The model under review builds one solid part; all positions refer to its coordinate system, in mm. A direction names the side the tool comes from. Give positions to 0.01 mm unless a question says otherwise; leave off trailing zeros. Order: outer loops, then holes, each group sorted by start corner. A loop starts at its lowest first (then second) coordinate and runs counter-clockwise, first axis right, second up.
```python
from build123d import *

# Parameters (mm, degrees)
SKETCH1_W                      = 225
SKETCH1_H                      = 150
SKETCH1_W_2                    = 5
SKETCH1_H_2                    = 80
BOSS_EXTRUDE1_DEPTH            = 5
CBORE_FOR_M5_SBHCS1_AT_2_COUNT = 2
CBORE_FOR_M5_SBHCS1_AT_2_PITCH = 210
CBORE_FOR_M5_SBHCS1_AT_3_COUNT = 2
CBORE_FOR_M5_SBHCS1_AT_3_PITCH = 135
CBORE_FOR_M5_SBHCS1_AT_4_COUNT = 2
CBORE_FOR_M5_SBHCS1_AT_4_PITCH = 249.649754656
FILLET1_R                      = 2


with BuildPart() as part:
    # Sketch1 → Boss-Extrude1 (new body)
    with BuildSketch(Plane(origin=(0, 0, 0), x_dir=(1, 0, 0), z_dir=(0, 1, 0))):
        Rectangle(SKETCH1_W, SKETCH1_H)
        with Locations((100, 0)):
            Rectangle(SKETCH1_W_2, SKETCH1_H_2, mode=Mode.SUBTRACT)
        with Locations((90, 0)):
            Rectangle(SKETCH1_W_2, SKETCH1_H_2, mode=Mode.SUBTRACT)
        with Locations((80, 0)):
            Rectangle(SKETCH1_W_2, SKETCH1_H_2, mode=Mode.SUBTRACT)
    extrude(amount=BOSS_EXTRUDE1_DEPTH)

    # Sketch3 → CBORE for M5 SBHCS1 (revolve, cut)
    with BuildSketch(Plane(origin=(-105, 5, -67.5), x_dir=(0, 0, 1), z_dir=(1, 0, 0))):
        Polygon((0, 0), (0, 5), (2.75, 5), (2.75, 2.75), (5.25, 2.75), (5.25, 0.025), (5.275, 0), align=None)
    cbore_for_m5_sbhcs1 = revolve(axis=Axis((-105, 11.35, -67.5), (0, -1, 0)), mode=Mode.SUBTRACT)

    # CBORE for M5 SBHCS1 at 2: CBORE for M5 SBHCS1 ×2
    with Locations(*[(i * CBORE_FOR_M5_SBHCS1_AT_2_PITCH, 0, 0) for i in range(1, CBORE_FOR_M5_SBHCS1_AT_2_COUNT)]):
        add(cbore_for_m5_sbhcs1, mode=Mode.SUBTRACT)

    # CBORE for M5 SBHCS1 at 3: CBORE for M5 SBHCS1 ×2
    with Locations(*[(0, 0, i * CBORE_FOR_M5_SBHCS1_AT_3_PITCH) for i in range(1, CBORE_FOR_M5_SBHCS1_AT_3_COUNT)]):
        add(cbore_for_m5_sbhcs1, mode=Mode.SUBTRACT)

    # CBORE for M5 SBHCS1 at 4: CBORE for M5 SBHCS1 ×2
    with Locations(*[Vector(0.8411784753765537, 0, 0.5407575913134988) * (i * CBORE_FOR_M5_SBHCS1_AT_4_PITCH) for i in range(1, CBORE_FOR_M5_SBHCS1_AT_4_COUNT)]):
        add(cbore_for_m5_sbhcs1, mode=Mode.SUBTRACT)

    # Fillet1
    fillet1_edges = [part.edges().sort_by_distance(p)[0] for p in [
        (-112.5, 5, 0),
        (0, 5, 75),
        (112.5, 5, 0),
        (0, 5, -75),
    ]]
    fillet(fillet1_edges, radius=FILLET1_R)


solid = part.part
```
Item 1: Take a section at C-C (y = 1.5). Give the boundary of the cut face in (x, z), and give its area (3 significant figures).
Values found:
outline: (-112.5, -75) - (112.5, -75) - (112.5, 75) - (-112.5, 75) - close; hole circle Ø5.5 at (-105, -67.5); hole circle Ø5.5 at (-105, 67.5); hole (77.5, -40) - (82.5, -40) - (82.5, 40) - (77.5, 40) - close; hole (87.5, -40) - (92.5, -40) - (92.5, 40) - (87.5, 40) - close; hole (97.5, -40) - (102.5, -40) - (102.5, 40) - (97.5, 40) - close; hole circle Ø5.5 at (105, -67.5); hole circle Ø5.5 at (105, 67.5)
area: 32,500 mm2
Item 2: Take a section at B-B (x = -105). Give the boundary of the cut face in (y, z) (3 decimals), and give its area (3 significant figures).
Values found:
outline: (0, -75) - (3, -75) arc R2 ccw to (5, -73) - (5, -72.775) - (4.975, -72.75) - (2.25, -72.75) - (2.25, -70.25) - (0, -70.25) - close; (0, -64.75) - (2.25, -64.75) - (2.25, -62.25) - (4.975, -62.25) - (5, -62.225) - (5, 62.225) - (4.975, 62.25) - (2.25, 62.25) - (2.25, 64.75) - (0, 64.75) - close; (0, 70.25) - (2.25, 70.25) - (2.25, 72.75) - (4.975, 72.75) - (5, 72.775) - (5, 73) arc R2 ccw to (3, 75) - (0, 75) - close
area: 666 mm2
Item 3: Take a section at A-A (z = 67.5). Give the boundary of the cut face in (x, y) (3 decimals).
Values found:
outline: (-112.5, 0) - (-107.75, 0) - (-107.75, 2.25) - (-110.25, 2.25) - (-110.25, 4.975) - (-110.275, 5) - (-110.5, 5) arc R2 ccw to (-112.5, 3) - close; (-102.25, 0) - (102.25, 0) - (102.25, 2.25) - (99.75, 2.25) - (99.75, 4.975) - (99.725, 5) - (-99.725, 5) - (-99.75, 4.975) - (-99.75, 2.25) - (-102.25, 2.25) - close; (107.75, 0) - (112.5, 0) - (112.5, 3) arc R2 ccw to (110.5, 5) - (110.275, 5) - (110.25, 4.975) - (110.25, 2.25) - (107.75, 2.25) - close
Item 4: For faces 3 (the flat face through (87.5, 2, 1)), 4 (the cylindrical face through (-108.55, 3.63, 63.63)), list the 3-axis set-ups (+Z, -Z, +X, -X, +Y, -Y) from which the entire face can be reached by the end or side of a thin tool; tool diameter is ignored.
Values found:
face 3: +Y, -Y
face 4: +Y
Item 5: Clearance check with flat-ended pins moving along their axes: pin 1 Ø5 at (x, z) = (-103.5, -70) entering from +Y; pin 2 Ø9.5 at (x, z) = (-105, -67.5) entering from +Y; pin 3 Ø1.5 at (x, y) = (73.5, 4) entering from -Z. State where each tip first meets the part, or that it passes through.
Values found:
pin 1: stops at y = 5
pin 2: stops at y = 2.25
pin 3: stops at z = -74.98
Item 6: For line 1 (X direction, y = 1.25, z = 67.5); line 2 (X direction, y = 3.25, z = -67.5); line 3 (X direction, y = 2.25, z = 7.5), list the stretches that pass through material, from the lowest coordinate up.
Values found:
line 1: x = -112.5 to -107.75, -102.25 to 102.25, 107.75 to 112.5
line 2: x = -112.48 to -110.25, -99.75 to 99.75, 110.25 to 112.48
line 3: x = -112.5 to 77.5, 82.5 to 87.5, 92.5 to 97.5, 102.5 to 112.5
Item 7: Draft analysis for pull direction Z (two halves, no side actions). For faces 1 (the flat face through (-2, 5, -1)), 2 (the flat face through (80, 2, 40)), state which applies: released by +Z, released by -Z, zero draft, split by the parting line, or undercut.
Values found:
face 1: zero draft
face 2: undercut
Item 8: Take a section at D-D (z = 17.5). Give the boundary of the cut face in (x, y).
Values found:
outline: (-112.5, 0) - (77.5, 0) - (77.5, 5) - (-110.5, 5) arc R2 ccw to (-112.5, 3) - close; (82.5, 0) - (87.5, 0) - (87.5, 5) - (82.5, 5) - close; (92.5, 0) - (97.5, 0) - (97.5, 5) - (92.5, 5) - close; (102.5, 0) - (112.5, 0) - (112.5, 3) arc R2 ccw to (110.5, 5) - (102.5, 5) - close
